Could you check a few things on this model? Use its own coordinates, in mm. Face numbers are marked on the shaded views. A direction names the side the tool comes from. Round coordinates to 2 decimals unless told otherwise and drop trailing zeros. Loops run counter-clockwise (first coordinate to the right, second up) from the corner with the lowest first, then second, coordinate; pieces in that order, holes last. Notation, with made-up numbers: (-20.5, 42.5) -> (6.5, 42.5) arc R19 cw to (6.5, 63.5) -> close; hole circle Ø3 at (-8, 48). An arc over 180 degrees is marked (long way). Write each question's results on one line, items separated by ' | '.
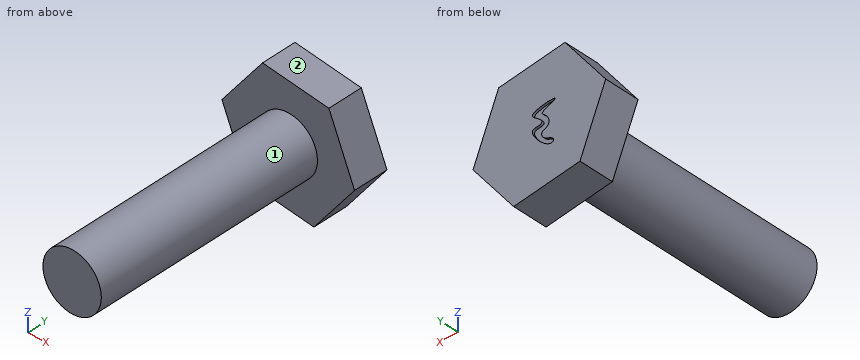
Autodesk Inventor part; units mm, degrees
ref_plane "YZ Plane" through (0, 0, 0) normal (1, 0, 0) x (0, 1, 0)
ref_plane "XZ Plane" through (0, 0, 0) normal (0, 1, 0) x (-1, 0, 0)
ref_plane "XY Plane" through (0, 0, 0) normal (0, 0, 1) x (1, 0, 0)
sketch "Sketch1" plane through (0, 0, 0) normal (0, 0, 1) x (1, 0, 0)
  line L0 (-17.9641, 7.8251) -> (-14.7891, 7.8251)
  line L1 (-14.7891, 7.8251) -> (-14.7891, -17.5749)
  line L2 (-14.7891, -17.5749) -> (-17.9641, -17.5749)
  line L3 (-17.9641, -17.5749) -> (-17.9641, 7.8251)
  point P0 (0, 0)
  dimension "d0" = 3.175
  dimension "d1" = 25.4
revolve "Revolution1" add sketch "Sketch1" angle 360 about axis through (-17.9641, -17.5749, 0) along (0, 1, 0)
sketch "Sketch2" plane through (-17.9641, 7.8251, 0) normal (0, 1, 0) x (1, 0, 0)
  circle A0 centre (0, 0) radius 3.175
  line L0 (-2.7933, -6.7141) -> (-7.2112, -0.938)
  line L1 (-7.2112, -0.938) -> (-4.418, 5.7761)
  line L2 (-4.418, 5.7761) -> (2.7933, 6.7141)
  line L3 (2.7933, 6.7141) -> (7.2112, 0.938)
  line L4 (7.2112, 0.938) -> (4.418, -5.7761)
  line L5 (4.418, -5.7761) -> (-2.7933, -6.7141)
  point P0 (17.9641, 0)
extrude "Extrusion1" add sketch "Sketch2" along normal blind 3.81 contours A0 | L0 L1 L2 L3 L4 L5
thread "Thread1"
sketch "Sketch3" plane through (-17.9641, 11.6351, 0) normal (0, 1, 0) x (1, 0, 0)
  spline S0 degree 5 poles (-1.6705, -1.7697) (-1.5087, -1.85) (-0.562, -1.832) (2.4108, -1.3359) (-1.0538, -0.5942) (-0.3082, 0.5963) (2.0933, -0.7076) (-1.4851, 3.8244) (-2.0876, 1.526) (-0.2865, 2.0954) (0.0858, 0.4541) (-1.2327, 0.9989) (-1.1868, -0.5585) (0.1138, -0.9114) (-0.367, -1.1465) (-1.6028, -1.5407) (-1.7853, -1.7128) (-1.6705, -1.7697) knots 0 0 0 0 0 0 0.118263 0.184405 0.277398 0.35545 0.432093 0.511849 0.589546 0.655005 0.725096 0.791185 0.859928 0.916088 1 1 1 1 1 1
  point P0 (17.9641, 0)
  point P1 (-0.2467, -0.2687)
  point P2 (-0.1215, 0.0477)
  point P3 (0.7392, 0.3)
  point P4 (-1.3859, 2.4418)
  point P5 (-1.4827, 2.0902)
  point P6 (-0.4576, 1.5038)
  point P7 (-0.3161, 0.9046)
  point P8 (-0.8855, 0.5658)
  point P9 (-0.8855, -0.3278)
  point P10 (-0.3187, -0.9153)
  point P11 (-0.8855, -1.3006)
extrude "Extrusion2" cut sketch "Sketch3" against normal blind 0.254
properties part number ".25 diameter 1'' bolt"
1) I want a section at B-B, the plane x = -14.25. Write out the boundary of the cut face in (y, z).
Model answer:
outline: (7.83, -5.51) -> (11.64, -5.51) -> (11.64, 5.87) -> (7.83, 5.87) -> close
2) I want a section at A-A, the plane y = -4.25. Write out the boundary of the cut face in (x, z) (3 decimals), plus the area to 3 significant figures.
Model answer:
outline: circle Ø6.35 at (-17.964, 0) | area: 31.7 mm2
3) I want a section at C-C, the plane z = 4. Write out the boundary of the cut face in (x, y), plus the area to 3 significant figures.
Model answer:
outline: (-22.83, 7.83) -> (-12.81, 7.83) -> (-12.81, 11.64) -> (-22.83, 11.64) -> close | area: 38.2 mm2
4) I'm going to push flat-ended pins straight in: pin 1 (5 mm diameter, centred on y = 8, z = -4, fed in from +X); pin 2 (2 mm diameter, centred on x = -16, y = -11, fed in from -Z); pin 3 (6 mm diameter, centred on y = -5.5, z = 1.5, fed in from +X). Where does each tip first touch, or does it pass through?
Model answer:
pin 1: stops at x = -11.18 | pin 2: stops at z = -3.03 | pin 3: stops at x = -14.79
5) For the marked faces 1 and 2, which set-ups out of +Z, -Z, +X, -X, +Y, -Y let a thin tool reach every point of the face, with its end or its side?
Model answer:
face 1: -Y | face 2: +Z, +X, +Y, -Y
6) I need wall thicknesses on line 1 (Y direction, x = -13, z = -2.25); line 2 (Y direction, x = -17.75, z = 1.5); line 3 (Z direction, x = -12.5, y = 9.5). Which ranges of each line are inside material? Lowest first, please.
Model answer:
line 1: y = 7.83 to 11.64 | line 2: y = -17.57 to 11.38 | line 3: z = -3.22 to 3.26
